from build123d import *

# Parameters (mm, degrees)
SKETCH2_R             = 85.5
BOSS_EXTRUDE1_DEPTH   = 5
SKETCH3_R             = 33
CUT_EXTRUDE1_DEPTH    = 122.018593613
SKETCH4_R             = 2.6
CUT_EXTRUDE2_DEPTH    = 122.018593613
CIRPATTERN3_COUNT     = 2
CIRPATTERN3_ANGLE     = 60
CIRPATTERN4_OUTLINE_R = 2.6
CIRPATTERN4_DEPTH     = 5


# Read off the part's stored shape, not the designer's step: CirPattern4
with BuildPart() as part:
    # Sketch2 → Boss-Extrude1 (new body)
    with BuildSketch(Plane.XY):
        Circle(SKETCH2_R)
    extrude(amount=BOSS_EXTRUDE1_DEPTH)

    # Sketch3 → Cut-Extrude1 (cut, through all)
    with BuildSketch(Plane.XY.offset(5)):
        with Locations((0, -23)):
            Circle(SKETCH3_R)
    extrude(amount=-CUT_EXTRUDE1_DEPTH, mode=Mode.SUBTRACT)

    # Sketch4 → Cut-Extrude2 (cut, through all)
    with BuildSketch(Plane.XY.offset(5)):
        with Locations((0, 67)):
            Circle(SKETCH4_R)
    cut_extrude2 = extrude(amount=-CUT_EXTRUDE2_DEPTH, mode=Mode.SUBTRACT)

    # CirPattern3: Cut-Extrude2 ×2 about axis
    cirpattern3_axis = Axis((0, 0, 5), (0, 0, 1))
    for i in range(1, CIRPATTERN3_COUNT):
        add(cut_extrude2.rotate(cirpattern3_axis, i * CIRPATTERN3_ANGLE / (CIRPATTERN3_COUNT - 1)), mode=Mode.SUBTRACT)

    # CirPattern4 outline → CirPattern4 (cut)
    with BuildSketch(Plane.XY):
        with Locations((58.023702054, 33.5)):
            Circle(CIRPATTERN4_OUTLINE_R)
    extrude(amount=CIRPATTERN4_DEPTH, mode=Mode.SUBTRACT)


solid = part.part
Can you work these out from the model? Positions are in its coordinate system, mm. Coordinates: 2 decimals unless noted, no trailing zeros. Write each loop counter-clockwise with the first axis right and the second up, starting at its lowest first coordinate (ties: lowest second). Pieces come first, ordered by that corner, then holes. Notation, with made-up numbers: (56, 54) - (68, 54) arc R14 ccw to (68, 75) - close; hole circle Ø1 at (59.25, 77). An arc over 180 degrees is marked (long way). Return JSON: item names as keys, results as strings. Group by question number.
Item 1: I'm going to push flat-ended pins straight in: pin 1 Ø1.5 at (x, z) = (-20, 1.5) entering from +Y; pin 2 Ø2 at (x, z) = (60.5, 2.5) entering from -Y; pin 3 Ø2 at (y, z) = (-35.5, 1) entering from +X. Where does each tip first touch, or does it pass through?
Item 2: Please list where these lines run through material, in increasing order: probe 1 along X at (y, z) = (-39, 1.5); probe 2 along Y at (x, z) = (-24.5, 2.75); probe 3 along Y at (x, z) = (-23, 0.9).
Item 3: If we section it at B-B (x = 30): Write out the boundary of the cut face in (y, z), then the cut area to 3 significant figures.
Item 4: If we section it at A-A (y = 33.5): Write out the boundary of the cut face in (x, z), then the cut area to 3 significant figures.
Item 5: If we section it at D-D (z = 1.5): Write out the boundary of the cut face in (x, y).
Item 6: We'd pull the mould along Y, two halves only. Please class faces 1 (the face through (-0.338, 69.578, 2.535)), 2 (the face through (81.552, 25.682, 2.465)), 3 (the face through (-1, 20, 0)): pulls with the +Y half, pulls with the -Y half, needs draft (parallel to the pull), parting line crosses it, or undercut.
Item 7: If we section it at C-C (y = 0): Write out the boundary of the cut face in (x, z).
Return value:
{
 "1": {"pin 1": "stops at y = 83.3", "pin 2": "stops at y = -61.4", "pin 3": "stops at x = 78.23"},
 "2": {"probe 1": "x = -76.09 to -28.86, 28.86 to 76.09", "probe 2": "y = -81.91 to -45.11, -0.89 to 81.91", "probe 3": "y = -82.35 to -46.66, 0.66 to 82.35"},
 "3": {"outline": "(-80.06, 0) - (-36.75, 0) - (-36.75, 5) - (-80.06, 5) - close; (-9.25, 0) - (80.06, 0) - (80.06, 5) - (-9.25, 5) - close", "area": "663 mm^2"},
 "4": {"outline": "(-78.66, 0) - (-60.62, 0) - (-60.62, 5) - (-78.66, 5) - close; (-55.42, 0) - (55.42, 0) - (55.42, 5) - (-55.42, 5) - close; (60.62, 0) - (78.66, 0) - (78.66, 5) - (60.62, 5) - close", "area": "735 mm^2"},
 "5": {"outline": "circle Ø171 at (0, 0); hole circle Ø5.2 at (-58.02, 33.5); hole circle Ø66 at (0, -23); hole circle Ø5.2 at (0, 67); hole circle Ø5.2 at (58.02, 33.5)"},
 "6": {"face 1": "undercut", "face 2": "parting line crosses it", "face 3": "needs draft"},
 "7": {"outline": "(-85.5, 0) - (-23.66, 0) - (-23.66, 5) - (-85.5, 5) - close; (23.66, 0) - (85.5, 0) - (85.5, 5) - (23.66, 5) - close"}
}
